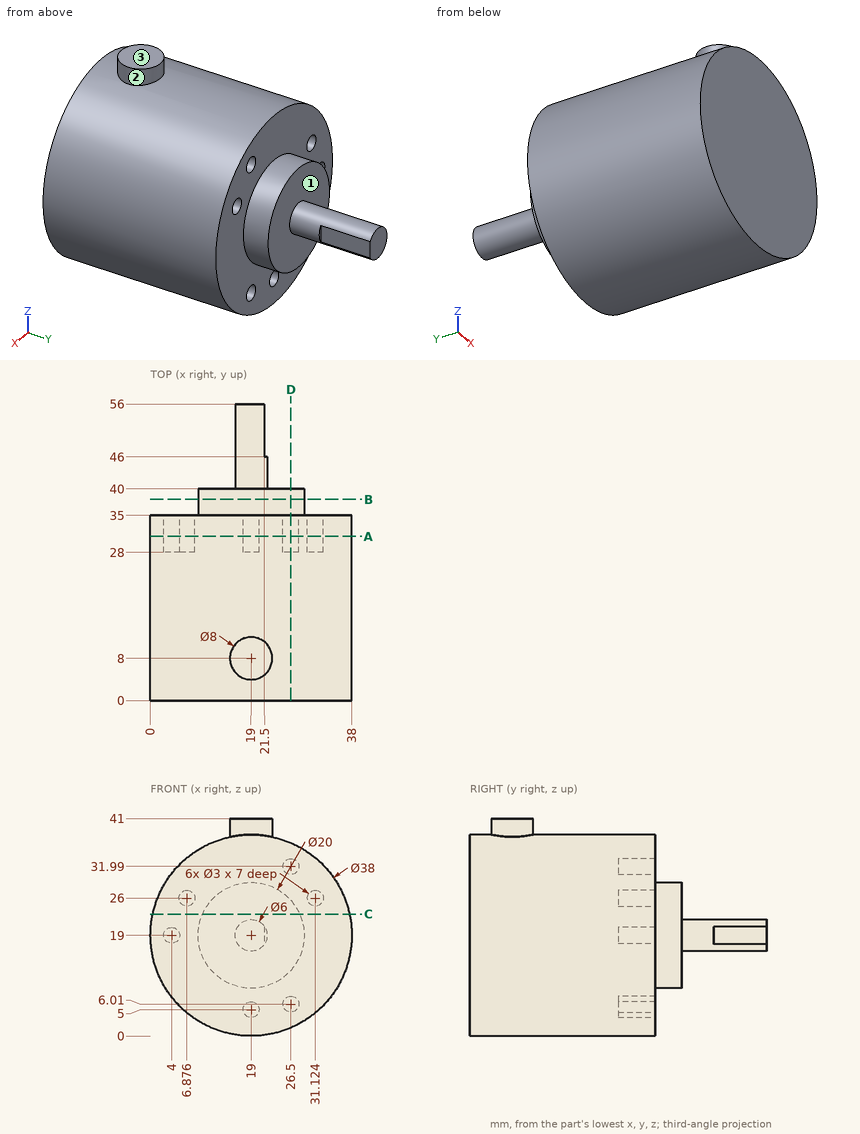
Could you check a few things on this drawing? It's one solid part, dimensions in mm from its lowest x, y, z. A direction names the side the tool comes from. Coordinates: 2 decimals unless noted, no trailing zeros. Order: outer loops, then holes, each group sorted by start corner. A loop starts at its lowest first (then second) coordinate and runs counter-clockwise, first axis right, second up. Notation, with made-up numbers: M -26,53 L -15,53 A26 cw -15,87 Z; hole C -32.75,77 d8. An arc over 180 degrees is marked long. Use a Markdown table: item, result. Add a question column.
Q1. I want a section at D-D on x = 26.5. List the corners of the cut face in (y, z) for me (1 decimal), then the cut area to 3 significant figures.
Q2. I want a section at C-C on z = 23. List the corners of the cut face in (x, y) for me (1 decimal), then the cut area to 3 significant figures.
Q3. I want a section at A-A on y = 31. List the corners of the cut face in (x, z) for me (1 decimal), then the cut area to 3 significant figures.
Q4. I want a section at B-B on y = 38. List the corners of the cut face in (x, z) for me.
Q5. If I drill on L1, parallel to X at y = 31, z = 19; L2, parallel to X at y = 29.75, z = 5 (1 decimal); L3, parallel to X at y = 31.75, z = 26 (1 decimal), over which ranges is the centre line in solid material (lowest first)?
Q6. I'm going to push flat-ended pins straight in: pin 1 (8 mm diameter, centred on x = 34, y = 31.5, fed in from -Z); pin 2 (4 mm diameter, centred on y = 32.5, z = 16, fed in from -X); pin 3 (1 mm diameter, centred on x = 22.5, y = 23, fed in from +Z); pin 4 (6 mm diameter, centred on x = 21, z = 15.5, fed in from +Y). Where does each tip first touch, or does it pass through?
Q7. Which directions (+Z, -Z, +X, -X, +Y, -Y) give clear straight access to the entire face, cutting with the end or side of a thin tool? Please do the marked faces 1, 2 and 3.
Checked values:
| question | item | result |
|---|---|---|
| 1 | outline | M 0,1.5 L 35,1.5 L 35,4.5 L 28,4.5 L 28,7.5 L 35,7.5 L 35,12.4 L 40,12.4 L 40,25.6 L 35,25.6 L 35,30.5 L 28,30.5 L 28,33.5 L 35,33.5 L 35,36.5 L 0,36.5 Z |
| 1 | area | 1,250 mm² |
| 2 | outline | M 0.4,0 L 37.6,0 L 37.6,35 L 28.2,35 L 28.2,40 L 9.8,40 L 9.8,35 L 0.4,35 Z |
| 2 | area | 1,390 mm² |
| 3 | outline | C 19,19 d38; hole C 4,19 d3; hole C 6.9,26 d3; hole C 19,5 d3; hole C 26.5,6 d3; hole C 26.5,32 d3; hole C 31.1,26 d3 |
| 3 | area | 1,090 mm² |
| 4 | outline | C 19,19 d20 |
| 5 | L1 | 0 to 2.5, 5.5 to 38 |
| 5 | L2 | 6.2 to 17.5, 20.5 to 25.4, 27.6 to 31.8 |
| 5 | L3 | 1.3 to 5.4, 8.4 to 29.6, 32.6 to 36.7 |
| 6 | pin 1 | z = 3.51 |
| 6 | pin 2 | x = 0.03 |
| 6 | pin 3 | z = 37.76 |
| 6 | pin 4 | y = 56 |
| 7 | face 1 | +Y |
| 7 | face 2 | +Z |
| 7 | face 3 | +Z, +X, -X, +Y, -Y |
